Autodesk Inventor part; units mm, degrees
ref_plane "C2_XY" through (0, 0, 0) normal (1, 0, 0) x (0, 0, -1)
ref_plane "C2_YZ" through (0, 0, 0) normal (0, 0, -1) x (0, 1, 0)
ref_plane "C2_ZX" through (0, 0, 0) normal (0, 1, 0) x (1, 0, 0)
sketch "Sketch_1" plane through (0, 0, 0) normal (0, 0, 1) x (1, 0, 0)
  line L0 (66, 0) -> (0, 0)
  line L1 (0, 0) -> (0, 3)
  line L2 (0, 3) -> (2.2517, 6.9)
  line L3 (2.2517, 6.9) -> (63.7483, 6.9)
  line L4 (63.7483, 6.9) -> (66, 3)
  line L5 (66, 3) -> (66, 0)
  line L6 (66, 0) -> (0, 0)
revolve "Revolution1" add sketch "Sketch_1" angle 360 about axis through (66, 0, 0) along (1, 0, 0)
sketch "Sketch_2" plane through (0, 0, 0) normal (1, 0, 0) x (0, 1, 0)
  line L0 (6.9, 6.9) -> (-6.9, 6.9)
  line L1 (-6.9, 6.9) -> (-6.9, -6.9)
  line L2 (-6.9, -6.9) -> (6.9, -6.9)
  line L3 (6.9, -6.9) -> (6.9, 6.9)
  line L4 (1.7321, 3) -> (-1.7321, 3)
  line L5 (-1.7321, 3) -> (-3.4641, 0)
  line L6 (-3.4641, 0) -> (-1.7321, -3)
  line L7 (-1.7321, -3) -> (1.7321, -3)
  line L8 (1.7321, -3) -> (3.4641, 0)
  line L9 (3.4641, 0) -> (1.7321, 3)
extrude "Extrusion1" cut sketch "Sketch_2" along normal blind 66
sketch "Sketch3" plane through (0, 0, 0) normal (-1, 0, 0) x (0, 0, 1)
  point P0 (0, 0)
hole "Hole1" at (0, 0, 0) direction (1, 0, 0) diameter 2.459 depth 8.2901 tip angle 120 countersink diameter 3 countersink angle 90
sketch "Sketch4" plane through (66, 0, 0) normal (1, 0, 0) x (0, 0, -1)
  point P0 (0, 0)
hole "Hole2" at (66, 0, 0) direction (-1, 0, 0) diameter 2.459 depth 8.2901 tip angle 120 countersink diameter 3 countersink angle 90
ref_plane "C2_XY" through (0, 0, 0) normal (1, 0, 0) x (0, 0, -1)
ref_plane "C2_YZ" through (0, 0, 0) normal (0, 0, -1) x (0, 1, 0)
ref_plane "C2_ZX" through (0, 0, 0) normal (0, 1, 0) x (1, 0, 0)
properties part number "ALSFB6-66" material "アルミニウム 2014-T4"
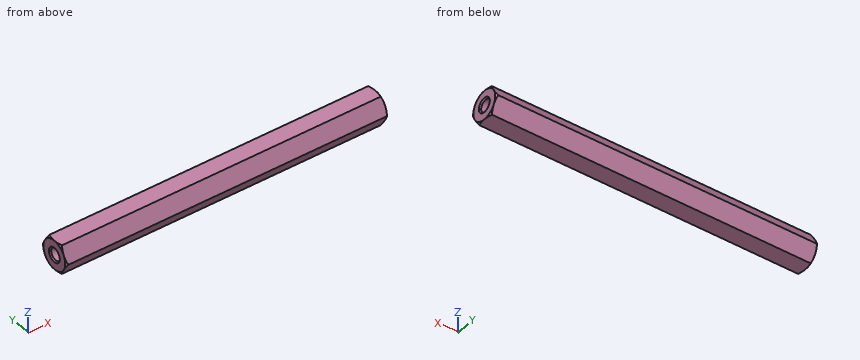
The listing builds one solid part. Answer for the finished solid, in the listing's coordinates (mm). Round coordinates to 2 decimals unless told otherwise and drop trailing zeros. Write each loop counter-clockwise with the first axis right and the second up, starting at its lowest first coordinate (ties: lowest second). Pieces come first, ordered by that corner, then holes. Notation, with made-up numbers: (68, -32.5) - (110, -32.5) arc R33 cw to (110, 6.5) - close; hole circle Ø8 at (43, 57.5). An arc over 180 degrees is marked (long way). Use one line per item in the form item = value. Start each with the question number.
Item 1: Find the intervals of material crossed by line 1 (Y direction, x = 63.5, z = 0); line 2 (Z direction, x = 59.5, y = 0); line 3 (Y direction, x = 19, z = -2.6), in increasing order. Write a range as [from, to].
Item 2: A flat-ended cylindrical pin translates along its axis: pin 1 Ø1.5 at (y, z) = (0, 0) entering from -X. Find the tip coordinate at first contact, or state that the pin passes through.
Item 3: A cutting plane is placed at A-A (x = 7). Write down the section's boundary in (y, z).
Item 4: A cutting plane is placed at B-B (x = 38.5). Write down the section's boundary in (y, z).
The answers:
q1.line_1 = [-3.46, -1.23], [1.23, 3.46]
q1.line_2 = [-3, -1.23], [1.23, 3]
q1.line_3 = [-1.96, 1.96]
q2.pin_1 = 8.57
q3.outline = (-3.46, 0) - (-1.73, -3) - (1.73, -3) - (3.46, 0) - (1.73, 3) - (-1.73, 3) - close; hole circle Ø2.46 at (0, 0)
q4.outline = (-3.46, 0) - (-1.73, -3) - (1.73, -3) - (3.46, 0) - (1.73, 3) - (-1.73, 3) - close
